from build123d import *

# Parameters (mm, degrees)
EXTRUDE_1_DEPTH     = 4
SKETCH_2_W          = 16.43
SKETCH_2_H          = 4
EXTRUDE_2_DEPTH     = 0.3
SKETCH_5_W          = 1.626393804
SKETCH_5_H          = 0.567965398
CUT_EXTRUDE_1_DEPTH = 0.02


with BuildPart() as part:
    # 草图1 → 凸台-拉伸1 (new body)
    with BuildSketch(Plane.XY):
        with BuildLine():
            Line((0, 0), (17.465, 0))
            ThreePointArc((17.465, 0), (18.101396103, -0.263603897), (18.365, -0.9))
            Line((18.365, -0.9), (18.365, -2.46))
            ThreePointArc((18.365, -2.46), (18.101396103, -3.096396103), (17.465, -3.36))
            Line((17.465, -3.36), (10.545, -3.36))
            Line((10.545, -3.36), (10.545, -3.46))
            Line((10.545, -3.46), (17.464999994, -3.46))
            ThreePointArc((17.464999994, -3.46), (18.172106779, -3.167106783), (18.465, -2.46))
            Line((18.465, -2.46), (18.465, -0.9))
            ThreePointArc((18.465, -0.9), (18.172106781, -0.192893219), (17.465, 0.1))
            Line((17.465, 0.1), (0, 0.1))
            Line((0, 0.1), (0, 0))
        make_face()
    extrude(amount=EXTRUDE_1_DEPTH)

    # 草图2 → 凸台-拉伸2 (add)
    with BuildSketch(Plane.XZ):
        with Locations((8.215, 2)):
            Rectangle(SKETCH_2_W, SKETCH_2_H)
    extrude(amount=EXTRUDE_2_DEPTH)

    # 草图5 → 切除-拉伸1 (cut)
    with BuildSketch(Plane.XZ.offset(3.46)):
        with Locations((11.358196902, 3.395)):
            Rectangle(SKETCH_5_W, SKETCH_5_H)
        with Locations((11.358196902, 2.465)):
            Rectangle(SKETCH_5_W, SKETCH_5_H)
        with Locations((11.358196902, 1.535)):
            Rectangle(SKETCH_5_W, SKETCH_5_H)
        with Locations((11.358196902, 0.605)):
            Rectangle(SKETCH_5_W, SKETCH_5_H)
    extrude(amount=-CUT_EXTRUDE_1_DEPTH, mode=Mode.SUBTRACT)


solid = part.part
Verification items for the finished model (mm, model axes). Round coordinates to 2 decimals unless told otherwise and drop trailing zeros. Write each loop counter-clockwise with the first axis right and the second up, starting at its lowest first coordinate (ties: lowest second). Pieces come first, ordered by that corner, then holes.
(1) Section check A-A (x = 13). Enter the section's corners in (y, z), plus the area to 3 significant figures.
Returned:
outline: (-3.46, 0) - (-3.36, 0) - (-3.36, 4) - (-3.46, 4) - close; (-0.3, 0) - (0.1, 0) - (0.1, 4) - (-0.3, 4) - close
area: 2.00 mm2
(2) Section check B-B (z = 2.95). Enter the section's corners in (x, y) (3 decimals).
Returned:
outline: (0, -0.3) - (16.43, -0.3) - (16.43, 0) - (17.465, 0) arc R0.9 cw to (18.365, -0.9) - (18.365, -2.46) arc R0.9 cw to (17.465, -3.36) - (10.545, -3.36) - (10.545, -3.46) - (17.465, -3.46) arc R1 ccw to (18.465, -2.46) - (18.465, -0.9) arc R1 ccw to (17.465, 0.1) - (0, 0.1) - close
(3) Section check C-C (x = 4.5). Enter the section's corners in (y, z), plus the area to 3 significant figures.
Returned:
outline: (-0.3, 0) - (0.1, 0) - (0.1, 4) - (-0.3, 4) - close
area: 1.60 mm2
(4) Mould release check, pull along Y, two halves, no side actions. Record for faces 1 (the flat face through (8, -0.3, 2)), 2 (the flat face through (9.2, -0.1, 4)), 3 (the flat face through (9, 0.1, 2)): pulls with the +Y half, pulls with the -Y half, needs draft (parallel to the pull), parting line crosses it, or undercut.
Returned:
face 1: undercut
face 2: needs draft
face 3: pulls with the +Y half
(5) Section check D-D (y = -1.3). Enter the section's corners in (x, z) (3 decimals), plus the area to 3 significant figures.
Returned:
outline: (18.365, 0) - (18.465, 0) - (18.465, 4) - (18.365, 4) - close
area: 0.400 mm2
(6) Material ranges on line 1 (Y direction, x = 2, z = 3.4); line 2 (X direction, y = -3.2, z = 0.65), recorded low to high.
Returned:
line 1: y = -0.3 to 0.1
line 2: x = 17.98 to 18.14
(7) Depth check by flat-ended pin: pin 1 Ø1.2 at (y, z) = (-1.5, 2) entering from -X (3 decimals); pin 2 Ø2 at (x, y) = (9.5, -1) entering from -Z; pin 3 Ø2 at (y, z) = (-2, 1) entering from -X (3 decimals). Enter the tip coordinate at first touch or a pass-through.
Returned:
pin 1: stops at x = 18.365
pin 2: stops at z = 0
pin 3: stops at x = 18.185
